Input: part model. Units: mm. Frame: model coordinates. Face numbers are marked on the shaded views. A direction names the side the tool comes from. Round coordinates to 2 decimals unless told otherwise and drop trailing zeros. One line per question, with ' | ' between items.
```python
from build123d import *

# Parameters (mm, degrees)
SKETCH055_R     = 1.45
PAD014_DEPTH    = 3
SKETCH060_R     = 0.15
POCKET028_DEPTH = 22
FILLET012_R     = 1.5


with BuildPart() as part:
    # Sketch055 → Pad014 (new body)
    with BuildSketch(Plane.XY):
        with BuildLine():
            add(Edge.make_bspline(
                [(150.875, 88.9625), (142.177266, 89.087472), (135.460331, 89.269548), (130.29585, 89.7876)],
                knots=[0, 0, 0, 0, 1, 1, 1, 1], degree=3))
            Line((130.29585, 89.7876), (128.95, 81.7125))
            Line((128.95, 81.7125), (143.625, 81.7125))
            Line((143.625, 81.7125), (143.625, 69.975))
            Line((143.625, 69.975), (150.975266, 70.587522))
            add(Edge.make_bspline(
                [(150.875, 88.9625), (150.875, 82.6662), (150.975266, 70.587522)],
                knots=[0, 0, 0, 1, 1, 1], degree=2))
        make_face()
        with Locations((147.25, 85.3375)):
            Circle(SKETCH055_R, mode=Mode.SUBTRACT)
    extrude(amount=PAD014_DEPTH)

    # Sketch060 → Pocket028 (cut)
    with BuildSketch(Plane.XY):
        with Locations((134.25, 85.3375)):
            Circle(SKETCH060_R)
        with Locations((147.25, 74.3375)):
            Circle(SKETCH060_R)
    extrude(amount=POCKET028_DEPTH, mode=Mode.SUBTRACT)

    # Fillet012
    fillet012_edges = [part.edges().sort_by_distance(p)[0] for p in [
        (150.875, 88.9625, 1.5),
    ]]
    fillet(fillet012_edges, radius=FILLET012_R)


with BuildPart() as part_1:
    # Body013 placement: moved
    add(part.part.moved(Location((0, 0, -6))))


solid = part_1.part
```
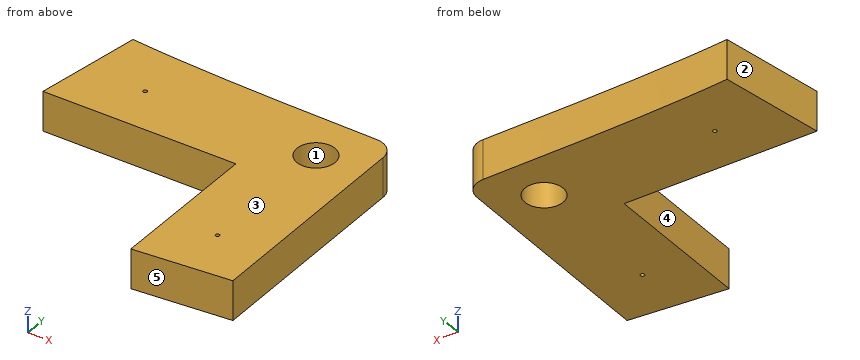
Item 1: Section query A-A, the plane z = -3.3. Give the number of separate pieces and of enclosed holes in the cut face, plus the area to 3 significant figures.
Report:
separate pieces: 1 | enclosed holes: 3 | area: 237 mm²
Item 2: Access query for the marked faces 4 and 5. Directions: +Z, -Z, +X, -X, +Y, -Y. A direction counts if a zero-diameter tool reaches every point of the face in a straight line with its end or side. Return the directions, or none.
Report:
face 4: +Z, -Z, -X, -Y | face 5: +Z, -Z, +X, -Y
Item 3: Mould query, pull axis X, two halves, no side actions, for the marked faces 1, 2 and 3. Classes: +X half, -X half, draft (parallel to the pull), parting line (faces both ways), or undercut.
Report:
face 1: undercut | face 2: -X half | face 3: draft
Item 4: First-contact query: pin 1 (1.5 mm diameter, centred on x = 134.5, z = -5, fed in from -Y); pin 2 (1.5 mm diameter, centred on y = 73.5, z = -5.5, fed in from +X); pin 3 (1.5 mm diameter, centred on y = 83.5, z = -3.5, fed in from -X). Flat tips, straight axial feed; report the tip coordinate or a pass-through.
Report:
pin 1: y = 81.71 | pin 2: x = 150.96 | pin 3: x = 129.12
Item 5: Line query: line 1 along Y through (x, z) = (147.25, -3.75); line 2 along X through (y, z) = (71.25, -5.3) (3 decimals); line 3 along X through (y, z) = (84.5, -3.15). Output: solid intervals per line, ascending. Write a range as from..to.
Report:
line 1: 70.28..74.19, 74.49..83.89, 86.79..89.02 | line 2: 143.625..150.97 | line 3: 129.41..146.07, 148.43..150.88
